from build123d import *

# Parameters (mm, degrees)
SKETCH1_W                = 71.1
SKETCH1_H                = 24.2
BOSS_EXTRUDE1_DEPTH      = 6
SKETCH2_W                = 71.1
SKETCH2_H                = 24.2
SKETCH2_W_2              = 2.5
SKETCH2_H_2              = 18.2
BOSS_EXTRUDE2_DEPTH      = 3
SKETCH3_W                = 80.1
SKETCH3_H                = 36.1
SKETCH3_R                = 1.55
BOSS_EXTRUDE3_DEPTH      = 1.8
SKETCH4_W                = 65
SKETCH4_H                = 15
BOSS_EXTRUDE4_DEPTH      = 0.001
BOSS_EXTRUDE4_DEPTH_BACK = 6
SKETCH5_W                = 41.7
SKETCH5_H                = 2.5
BOSS_EXTRUDE5_DEPTH      = 2.5
SKETCH6_W                = 0.6
SKETCH6_H                = 0.6
SKETCH6_W_2              = 0.52
BOSS_EXTRUDE6_DEPTH      = 6


with BuildPart() as part:
    # Sketch1 → Boss-Extrude1 (new body)
    with BuildSketch(Plane(origin=(0, 0, 0), x_dir=(1, 0, 0), z_dir=(0, 1, 0))):
        Rectangle(SKETCH1_W, SKETCH1_H)
    extrude(amount=BOSS_EXTRUDE1_DEPTH)

    # Sketch2 → Boss-Extrude2 (add)
    with BuildSketch(Plane.XZ):
        Rectangle(SKETCH2_W, SKETCH2_H)
        with Locations((-36.8, 0)):
            Rectangle(SKETCH2_W_2, SKETCH2_H_2)
    extrude(amount=BOSS_EXTRUDE2_DEPTH)

    # Sketch3 → Boss-Extrude3 (add)
    with BuildSketch(Plane.XZ.offset(3)):
        Rectangle(SKETCH3_W, SKETCH3_H)
        with Locations((-37.55, -15.55)):
            Circle(SKETCH3_R, mode=Mode.SUBTRACT)
        with Locations((37.55, -15.55)):
            Circle(SKETCH3_R, mode=Mode.SUBTRACT)
        with Locations((37.55, 15.55)):
            Circle(SKETCH3_R, mode=Mode.SUBTRACT)
        with Locations((-37.55, 15.55)):
            Circle(SKETCH3_R, mode=Mode.SUBTRACT)
    extrude(amount=BOSS_EXTRUDE3_DEPTH)

    # Sketch4 → Boss-Extrude4 (add, two sides)
    with BuildSketch(Plane(origin=(0, 6, 0), x_dir=(1, 0, 0), z_dir=(0, 1, 0))) as boss_extrude4_sk:
        Rectangle(SKETCH4_W, SKETCH4_H)
    extrude(amount=BOSS_EXTRUDE4_DEPTH)
    extrude(boss_extrude4_sk.sketch, amount=-BOSS_EXTRUDE4_DEPTH_BACK)

    # Sketch5 → Boss-Extrude5 (add)
    with BuildSketch(Plane.XZ.offset(4.8)):
        with Locations((12.2, 15.3)):
            Rectangle(SKETCH5_W, SKETCH5_H)
    extrude(amount=BOSS_EXTRUDE5_DEPTH)

    # Sketch6 → Boss-Extrude6 (add)
    with BuildSketch(Plane.XZ.offset(7.3)):
        with Locations((32.25, 15.292216916)):
            Rectangle(SKETCH6_W, SKETCH6_H)
        with Locations((29.61, 15.292216916)):
            Rectangle(SKETCH6_W_2, SKETCH6_H)
        with Locations((26.89, 15.292216916)):
            Rectangle(SKETCH6_W, SKETCH6_H)
        with Locations((24.21, 15.292216916)):
            Rectangle(SKETCH6_W, SKETCH6_H)
        with Locations((21.53, 15.292216916)):
            Rectangle(SKETCH6_W, SKETCH6_H)
        with Locations((18.85, 15.292216916)):
            Rectangle(SKETCH6_W, SKETCH6_H)
        with Locations((16.17, 15.292216916)):
            Rectangle(SKETCH6_W, SKETCH6_H)
        with Locations((13.49, 15.292216916)):
            Rectangle(SKETCH6_W, SKETCH6_H)
        with Locations((10.81, 15.292216916)):
            Rectangle(SKETCH6_W, SKETCH6_H)
        with Locations((8.13, 15.292216916)):
            Rectangle(SKETCH6_W, SKETCH6_H)
        with Locations((5.45, 15.292216916)):
            Rectangle(SKETCH6_W, SKETCH6_H)
        with Locations((2.77, 15.292216916)):
            Rectangle(SKETCH6_W, SKETCH6_H)
        with Locations((-7.95, 15.292216916)):
            Rectangle(SKETCH6_W, SKETCH6_H)
        with Locations((-5.27, 15.292216916)):
            Rectangle(SKETCH6_W, SKETCH6_H)
        with Locations((0.09, 15.292216916)):
            Rectangle(SKETCH6_W, SKETCH6_H)
        with Locations((-2.59, 15.292216916)):
            Rectangle(SKETCH6_W, SKETCH6_H)
    extrude(amount=BOSS_EXTRUDE6_DEPTH)


solid = part.part
Build history of the part. All positions in model axes, mm. A direction names the side the tool comes from. Coordinates: 2 decimals unless noted, no trailing zeros. Order: outer loops, then holes, each group sorted by start corner. A loop starts at its lowest first (then second) coordinate and runs counter-clockwise, first axis right, second up. Notation, with made-up numbers: (8, 11) - (54, 11) arc R19 cw to (54, 45) - close; hole circle Ø3 at (43, 12.25). An arc over 180 degrees is marked (long way). Write item = value, one per line. Start each with the question number.
1) Wall check: line 1 along Z through (x, y) = (-37.55, -4.3); line 2 along Y through (x, z) = (-9.5, -6.5); line 3 along Z through (x, y) = (27.5, 3.75). Give the ranges that are in metal, low to high. Write a range as from..to.
2) Saw through at C-C on y = -1.5. Write the cut outline in (x, z), then the cut area to 3 significant figures.
3) 3-axis set-ups, long thin cutter, end or side, ignore diameter. For faces 1 (the face through (-38.05, -1, 0)), 2 (the face through (0, 6, -8)), 3 (the face through (12, -6, 14.05)), 4 (the face through (33.05, -6, 15)), 5 (the face through (0, 2, -12.1)): which of +Z, -Z, +X, -X, +Y, -Y reach the whole face in a straight line?
4) Saw through at D-D on y = -9.75. Count the separate pieces of the cut face and the enclosed holes in it, then the cut area to 3 significant figures.
5) Flat gauge pins, fed straight in: pin 1 Ø6 at (x, z) = (25.5, 4) entering from -Y; pin 2 Ø0.5 at (y, z) = (-10.5, 15.5) entering from -X; pin 3 Ø1.5 at (y, z) = (-1, 3.5) entering from -X. Where does each tip first touch, or does it go through?
6) Two-plate mould, pull along Z, no slides. Class faces 6 (the face through (36, -3.9, 15.6)), 7 (the face through (-1, -4, 18.05)), 8 (the face through (-8.65, -6, 15)), 9 (the face through (-37, -1, -9.1)): pulls with the +Z half, pulls with the -Z half, needs draft (parallel to the pull), parting line crosses it, or undercut.
7) Saw through at A-A on x = 37.55. Write the cut outline in (y, z).
From the geometry:
q1.line_1 = -18.05..-17.1, -14..14, 17.1..18.05
q1.line_2 = -4.8..6
q1.line_3 = -12.1..12.1
q2.outline = (-38.05, -9.1) - (-35.55, -9.1) - (-35.55, -12.1) - (35.55, -12.1) - (35.55, 12.1) - (-35.55, 12.1) - (-35.55, 9.1) - (-38.05, 9.1) - close
q2.area = 1,770 mm^2
q3.face_1 = +Z, -Z, -X, +Y
q3.face_2 = +Z, -Z, +X, -X, +Y
q3.face_3 = -Z, +X, -X, -Y
q3.face_4 = +Z, -Z, +X, -Y
q3.face_5 = -Z, +X, -X, +Y
q4.separate_pieces = 16
q4.enclosed_holes = 0
q4.area = 5.71 mm^2
q5.pin_1 = -4.8
q5.pin_2 = -8.25
q5.pin_3 = -38.05
q6.face_6 = undercut
q6.face_7 = pulls with the +Z half
q6.face_8 = needs draft
q6.face_9 = pulls with the -Z half
q7.outline = (-4.8, -18.05) - (-3, -18.05) - (-3, -17.1) - (-4.8, -17.1) - close; (-4.8, -14) - (-3, -14) - (-3, 14) - (-4.8, 14) - close; (-4.8, 17.1) - (-3, 17.1) - (-3, 18.05) - (-4.8, 18.05) - close
